Part model, mm, in its own coordinate system. A direction names the side the tool comes from. Give positions to 0.01 mm unless a question says otherwise; leave off trailing zeros. Order: outer loops, then holes, each group sorted by start corner. A loop starts at its lowest first (then second) coordinate and runs counter-clockwise, first axis right, second up. Notation, with made-up numbers: (-36.5, -16) - (17.5, -16) arc R33 cw to (17.5, 22) - close; hole circle Ø8 at (41, 76.5). An arc over 180 degrees is marked (long way). Use one line per item in the form item = value. Start each with the question number.
1. Band-saw the part on B-B, the plane z = 10.5. List the corners of the cut face in (x, y).
2. Pull direction Z, two halves, no side cores. Call faces 3 (the face through (1.3, -1.3, 14)), 4 (the face through (0, 2, 12)), 5 (the face through (0, 0, 0)), 6 (the face through (1, -2, 11)): +Z half, -Z half, draft (parallel to the pull), parting line (faces both ways), or undercut.
3. Tool access for faces 1 (the face through (2.86, 0.9, 6.9)), 2 (the face through (0, 0, 6)): list every direction of +Z, -Z, +X, -X, +Y, -Y with a clear straight run to the whole face (end or side of a thin tool).
4. Pin check, flat tips, straight feed: P1, Ø1.6, axis at x = 0, z = 11, coming from the +Y side; P2, Ø2.5, axis at x = 0, y = 0, coming from the +Z side. Stop position of each tip, or through.
5. Band-saw the part on A-A, the plane x = 0. List the corners of the cut face in (y, z), plus the area to 3 significant figures.
6. Band-saw the part on D-D, the plane y = 2.5. List the corners of the cut face in (x, z), plus the area to 3 significant figures.
7. Drill centre lines: line 1 (Z direction, x = 0, y = 2.3); line 2 (X direction, y = 1.85, z = 11); line 3 (X direction, y = 2.1, z = 11). Where is each one in solid material? Low to high.
8. Band-saw the part on C-C, the plane y = 0. List the corners of the cut face in (x, z).
from build123d import *

# Parameters (mm, degrees)
SKETCH002_R  = 1
PAD001_DEPTH = 5
SKETCH_R     = 3
PAD_DEPTH    = 14
SKETCH001_R  = 1.5
POCKET_DEPTH = 8


with BuildPart() as pad001:
    # Sketch002 → Pad001 (new body, symmetric)
    with BuildSketch(Plane.XZ):
        with Locations((0, 11)):
            Circle(SKETCH002_R)
    extrude(amount=PAD001_DEPTH, both=True)


with BuildPart() as cut:
    # Sketch → Pad (new body)
    with BuildSketch(Plane.XY):
        Circle(SKETCH_R)
    extrude(amount=PAD_DEPTH)

    # Sketch001 → Pocket (cut)
    with BuildSketch(Plane.XY.offset(14)):
        Circle(SKETCH001_R)
    extrude(amount=-POCKET_DEPTH, mode=Mode.SUBTRACT)

    # Cut: cut Pad001
    add(pad001.part, mode=Mode.SUBTRACT)


solid = cut.part
From the geometry:
q1.outline = (-0.87, -2.87) - (-0.87, -1.22) arc R1.5 cw to (-0.87, 1.22) - (-0.87, 2.87) arc R3 ccw to start; (0.87, -2.87) arc R3 ccw to (0.87, 2.87) - (0.87, 1.22) arc R1.5 cw to (0.87, -1.22) - close
q2.face_3 = +Z half
q2.face_4 = undercut
q2.face_5 = -Z half
q2.face_6 = undercut
q3.face_1 = +Z, -Z
q3.face_2 = +Z
q4.P1 = through
q4.P2 = 6
q5.outline = (-3, 0) - (3, 0) - (3, 10) - (1.5, 10) - (1.5, 6) - (-1.5, 6) - (-1.5, 10) - (-3, 10) - close; (-3, 12) - (-1.5, 12) - (-1.5, 14) - (-3, 14) - close; (1.5, 12) - (3, 12) - (3, 14) - (1.5, 14) - close
q5.area = 54.0 mm²
q6.outline = (-1.66, 0) - (1.66, 0) - (1.66, 14) - (-1.66, 14) - close; hole circle Ø2 at (0, 11)
q6.area = 43.3 mm²
q7.line_1 = 0 to 10, 12 to 14
q7.line_2 = -2.36 to -1, 1 to 2.36
q7.line_3 = -2.14 to -1, 1 to 2.14
q8.outline = (-3, 0) - (3, 0) - (3, 14) - (1.5, 14) - (1.5, 6) - (-1.5, 6) - (-1.5, 14) - (-3, 14) - close
